Geometry check sheet. Reference: the model listing, model coordinates, mm. A direction names the side the tool comes from. Coordinates: 2 decimals unless noted, no trailing zeros. Order: outer loops, then holes, each group sorted by start corner. A loop starts at its lowest first (then second) coordinate and runs counter-clockwise, first axis right, second up. Notation, with made-up numbers: (-23.75, -20.75) - (-2.75, -20.75) arc R16 ccw to (-2.75, 6.25) - close; hole circle Ø10 at (67, -13.75). An arc over 180 degrees is marked (long way). Use CSV: the item, a comma, the result in double quotes. Start each with the question number.
1) Draft check along X on faces 6 (the cylindrical face through (394.297, -2.958, 123.986)), 7 (the cylindrical face through (294.297, -2.958, 86.014)), 8 (the cylindrical face through (65.27, -2.96, 98.74)). Enter one of: released by +X, released by -X, zero draft, split by the parting line, or undercut.
2) Sectioned sample at A-A, the plane x = 175. Record the cut outline in (y, z), and give its area (3 significant figures).
3) Sectioned sample at C-C, the plane z = 223. Record the cut outline in (x, y), and give its area (3 significant figures).
4) Tool access check on faces 1 (the cylindrical face through (176.014, -2.958, 85.703)), 2 (the cylindrical face through (174.64, -2.96, 372.81)), 3 (the cylindrical face through (306.014, -2.958, 124.297)), 4 (the flat face through (114.52, -2.96, 275.78)), 5 (the cylindrical face through (195.048, -2.958, 416.284)). Record the directions out of +Z, -Z, +X, -X, +Y, -Y that give a thin tool (end or side, any length) a straight path to the whole face; none if there is none.
5) Thickness scan on probe 1 along Z at (x, y) = (169, -1.75); probe 2 along Z at (x, y) = (328.5, -4.25); probe 3 along Z at (x, y) = (206.5, -1.75). Record the ranges inside material, lowest first. Write a range as [from, to].
6) Depth check by flat-ended pin: P1, Ø1.8, axis at x = 8, y = -2.5, coming from the +Z side; P2, Ø3, axis at y = -2, z = 314.5, coming from the +X side; P3, Ø2, axis at x = 280.5, y = -1.5, coming from the -Z side; P4, Ø1.8, axis at x = 357, y = -2, coming from the +Z side. Enter the tip coordinate at first touch or a pass-through.
7) Sectioned sample at B-B, the plane x = 363.5. Record the cut outline in (y, z), and give its area (3 significant figures).
from build123d import *

# Parameters (mm, degrees)
F1_DEPTH = 6
F2_R     = 20
F4_W     = 58.9145278931
F4_H     = 17
F5_DEPTH = 25


with BuildPart() as f1:
    # F0 (on Front) → F1 (new body)
    with BuildSketch(Plane.XZ):
        with BuildLine():
            Line((0, 80), (0, 0))
            Line((0, 0), (400, 0))
            Line((400, 0), (400, 110))
            ThreePointArc((400, 110), (394.1421356237, 124.1421356237), (380, 130))
            Line((380, 130), (320, 130))
            ThreePointArc((320, 130), (305.8578643763, 124.1421356237), (300, 110))
            Line((300, 110), (300, 100))
            ThreePointArc((300, 100), (294.1421356237, 85.8578643763), (280, 80))
            Line((280, 80), (190, 80))
            ThreePointArc((190, 80), (175.8578643763, 85.8578643763), (170, 100))
            Line((170, 100), (170, 360))
            ThreePointArc((170, 360), (175.8578643763, 374.1421356237), (190, 380))
            Line((190, 380), (212, 380))
            Line((212, 380), (202.2308922809, 406.8404028665))
            ThreePointArc((202.2308922809, 406.8404028665), (194.9085685922, 416.3830408858), (183.4370398652, 420))
            Line((183.4370398652, 420), (156.7331660644, 420))
            ThreePointArc((156.7331660644, 420), (143.8774138707, 415.3208888624), (137.0370110042, 403.4729635533))
            Line((137.0370110042, 403.4729635533), (91.3652335031, 144.455442142))
            ThreePointArc((91.3652335031, 144.455442142), (64.6876623237, 98.2485334367), (14.5502287682, 80))
            Line((14.5502287682, 80), (0, 80))
        make_face()
    extrude(amount=F1_DEPTH)

    # F2
    f2_edges = [f1.edges().sort_by_distance(p)[0] for p in [
        (212, -3, 380),
    ]]
    fillet(f2_edges, radius=F2_R)

    # F4 (on face) → F5 (cut)
    with BuildSketch(Plane.XZ.offset(6)):
        with Locations((169.4572639465, 238.5)):
            Rectangle(F4_W, F4_H)
    extrude(amount=-F5_DEPTH, mode=Mode.SUBTRACT)


solid = f1.part
Evaluation:
1,face 6,"released by +X"
1,face 7,"undercut"
1,face 8,"released by -X"
2,outline,"(-6, 0) - (0, 0) - (0, 86.77) - (-6, 86.77) - close; (-6, 373.23) - (0, 373.23) - (0, 420) - (-6, 420) - close"
2,area,"801 mm²"
3,outline,"(105.21, -6) - (170, -6) - (170, 0) - (105.21, 0) - close"
3,area,"389 mm²"
4,face 1,"+Y, -Y"
4,face 2,"+X, +Y, -Y"
4,face 3,"+Z, +Y, -Y"
4,face 4,"+Z, -X, +Y, -Y"
4,face 5,"+Z, +X, +Y, -Y"
5,probe 1,"[0, 230], [247, 420]"
5,probe 2,"[0, 130]"
5,probe 3,"[0, 80]"
6,P1,"z = 80"
6,P2,"x = 170"
6,P3,"z = 0"
6,P4,"z = 130"
7,outline,"(-6, 0) - (0, 0) - (0, 130) - (-6, 130) - close"
7,area,"780 mm²"
